Check sheet for the drawn part. Datum: minimum x, y, z corner. Units: mm. A direction names the side the tool comes from. Give positions to 0.01 mm unless a question says otherwise; leave off trailing zeros. Loops run counter-clockwise (first coordinate to the right, second up) from the corner with the lowest first, then second, coordinate; pieces in that order, holes last.
1. Cross-section at C-C, the plane x = 57.5. Record the cut outline in (y, z).
2. Tool access check on the marked faces 1 and 2. Record the directions out of +Z, -Z, +X, -X, +Y, -Y that give a thin tool (end or side, any length) a straight path to the whole face; none if there is none.
3. Go/stop test with a flat-tipped pin: pin 1 Ø4 at (x, y) = (53, 13) entering from +Z. Record where the tip stops, or that it passes through.
4. Release check for a two-part mould opening along X. For the marked faces 3, 4, 5 and 6 record: +X half, -X half, draft (parallel to the pull), parting line (faces both ways), or undercut.
5. Cross-section at A-A, the plane z = 58. Record the cut outline in (x, y).
6. Material ranges on L1, parallel to X at y = 10.5, z = 63; L2, parallel to Z at x = 39, y = 21, recorded low to high.
7. Cross-section at B-B, the plane y = 2. Record the cut outline in (x, z), plus the area to 3 significant figures.
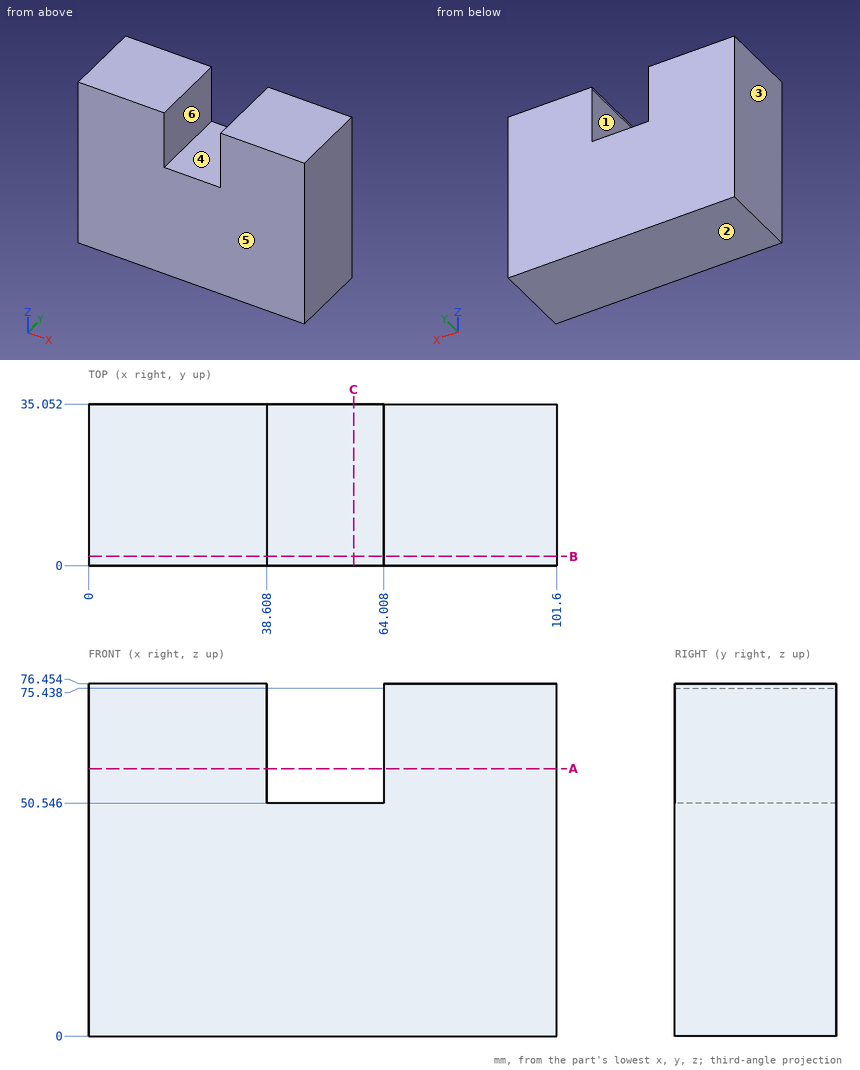
Result:
1. outline: (0, 0) - (35.05, 0) - (35.05, 50.55) - (0, 50.55) - close
2. face 1: +Z, +Y, -Y
2. face 2: -Z, +X, -X, +Y, -Y
3. pin 1: stops at z = 50.55
4. face 3: -X half
4. face 4: undercut
4. face 5: draft
4. face 6: undercut
5. outline: (0, 0) - (38.61, 0) - (38.61, 35.05) - (0, 35.05) - close; (64.01, 0) - (101.6, 0) - (101.6, 35.05) - (64.01, 35.05) - close
6. L1: x = 0 to 38.61, 64.01 to 101.6
6. L2: z = 0 to 50.55
7. outline: (0, 0) - (101.6, 0) - (101.6, 76.45) - (64.01, 76.45) - (64.01, 50.55) - (38.61, 50.55) - (38.61, 76.45) - (0, 76.45) - close
7. area: 7,110 mm2
